Part model, mm, in its own coordinate system. A direction names the side the tool comes from. Coordinates: 2 decimals unless noted, no trailing zeros. Write each loop counter-clockwise with the first axis right and the second up, starting at its lowest first coordinate (ties: lowest second). Pieces come first, ordered by that corner, then holes. Notation, with made-up numbers: (-35.5, 84.5) - (9.5, 84.5) arc R20 cw to (9.5, 103.5) - close; hole circle Ø1 at (9.25, 12.5). An arc over 180 degrees is marked (long way). Write each question's results on one line, items separated by ' | '.
from build123d import *

# Parameters (mm, degrees)
F1_DEPTH = 10
F2_W     = 10
F2_H     = 6
F3_DEPTH = 5
F2_R     = 2.6
F4_DEPTH = 3
F5_R     = 2.6
F6_DEPTH = 3
F7_DEPTH = 5


with BuildPart() as f1:
    # F0 (on Front) → F1 (new body, symmetric)
    with BuildSketch(Plane.XZ):
        Polygon((90, 0), (-90, 0), (-90, -3), (-70, -3), (-45.843204, -140), (45.843204, -140), (70, -3), (90, -3), align=None)
        Polygon((-66.601066, -5), (-66.95372, -3), (-64.95372, -3), (66.95372, -3), (43.678559, -135), (43.325905, -137), (42.031213, -137), (-43.325905, -137), align=None, mode=Mode.SUBTRACT)
    extrude(amount=F1_DEPTH, both=True)

    # F2 (on face) → F3 (join)
    with BuildSketch(Plane.XY):
        with Locations((-60, 0)):
            Rectangle(F2_W, F2_H)
        with Locations((60, 0)):
            Rectangle(F2_W, F2_H)
    extrude(amount=F3_DEPTH)

    # F2 (on face) → F4 (cut, through all)
    with BuildSketch(Plane.XY):
        with Locations((-80, 0)):
            Circle(F2_R)
        with Locations((80, 0)):
            Circle(F2_R)
    extrude(amount=-F4_DEPTH, mode=Mode.SUBTRACT)

    # F5 (on face) → F6 (cut, through all)
    with BuildSketch(Plane.XY.offset(-137)):
        with Locations((-23.325905, 0)):
            Circle(F5_R)
        with Locations((22.031213, 0)):
            Circle(F5_R)
    extrude(amount=-F6_DEPTH, mode=Mode.SUBTRACT)

    # F0 (on Front) → F7 (join, symmetric)
    with BuildSketch(Plane.XZ):
        Polygon((-64.95372, -3), (-66.95372, -3), (-66.601066, -5), (42.031213, -137), (43.325905, -137), (43.678559, -135), align=None)
    extrude(amount=F7_DEPTH, both=True)


solid = f1.part
(1) Flat gauge pins, fed straight in: P1, Ø10, axis at x = -83, y = -2.5, coming from the -Z side; P2, Ø2.5, axis at y = 1, z = 3, coming from the +X side; P3, Ø10, axis at x = -34.5, y = 4, coming from the +Z side. Where does each tip first touch, or does it go through?
Return value:
P1: stops at z = -3 | P2: stops at x = 65 | P3: stops at z = 0
(2) Saw through at A-A on y = -7.5. Write the cut outline in (x, z), then the cut area to 3 significant figures.
Return value:
outline: (-90, -3) - (-70, -3) - (-45.84, -140) - (45.84, -140) - (70, -3) - (90, -3) - (90, 0) - (-90, 0) - close; hole (-66.95, -3) - (-43.33, -137) - (43.33, -137) - (66.95, -3) - close | area: 1,630 mm^2
(3) 3-axis set-ups, long thin cutter, end or side, ignore diameter. For faces 1 (the flat face through (-55, 0, 2)), 2 (the flat face through (-65, 0, 2)), 3 (the flat face through (82, -2, -3)), 4 (the cylindrical face through (19.434, 0.114, -138.479)), 5 (the flat face through (-60, -3, 2)): which of +Z, -Z, +X, -X, +Y, -Y reach the whole face in a straight line?
Return value:
face 1: +Z, +Y, -Y | face 2: +Z, -X, +Y, -Y | face 3: -Z, +X, +Y, -Y | face 4: -Z | face 5: +Z, +X, -X, -Y
(4) Two-plate mould, pull along Z, no slides. Class faces 6 (the flat face through (-1, 0, -140)), 7 (the flat face through (-12, 5, -70)), 8 (the flat face through (-12, -5, -70)), 9 (the cylindrical face through (-82.6, 0.1, -1.5)): released by +Z, released by -Z, zero draft, split by the parting line, or undercut.
Return value:
face 6: released by -Z | face 7: undercut | face 8: undercut | face 9: zero draft
(5) Saw through at D-D on x = 6.5. Write the cut outline in (y, z).
Return value:
outline: (-10, -140) - (10, -140) - (10, -137) - (-10, -137) - close; (-10, -3) - (10, -3) - (10, 0) - (-10, 0) - close; (-5, -93.83) - (5, -93.83) - (5, -89.82) - (-5, -89.82) - close
(6) Wall check: line 1 (Y direction, x = 80, z = -1); line 2 (Z direction, x = -27.5, y = -4.5); line 3 (X direction, y = -3.5, z = -98). Give the ranges that are in metal, low to high. Write a range as from..to.
Return value:
line 1: y = -10..-2.6, 2.6..10 | line 2: z = -140..-137, -52.51..-48.51, -3..0 | line 3: x = -53.25..-50.2, 9.94..13.23, 50.2..53.25
(7) Saw through at C-C on z = -129.5. Write the cut outline in (x, y).
Return value:
outline: (-47.69, -10) - (-44.65, -10) - (-44.65, 10) - (-47.69, 10) - close; (35.86, -5) - (39.15, -5) - (39.15, 5) - (35.86, 5) - close; (44.65, -10) - (47.69, -10) - (47.69, 10) - (44.65, 10) - close
(8) Saw through at B-B on x = 80. Write the cut outline in (y, z).
Return value:
outline: (-10, -3) - (-2.6, -3) - (-2.6, 0) - (-10, 0) - close; (2.6, -3) - (10, -3) - (10, 0) - (2.6, 0) - close
